Here's the drawing with two shaded views (mm, measured from the low corner). I have some questions. Coordinates: 2 decimals unless noted, no trailing zeros. Order: outer loops, then holes, each group sorted by start corner. A loop starts at its lowest first (then second) coordinate and runs counter-clockwise, first axis right, second up. Notation, with made-up numbers: (16.5, -34) -> (23.5, -34) arc R28 ccw to (23.5, 1) -> close; hole circle Ø10 at (31.5, 1.5). An arc over 180 degrees is marked (long way). Write item = value, one per line.
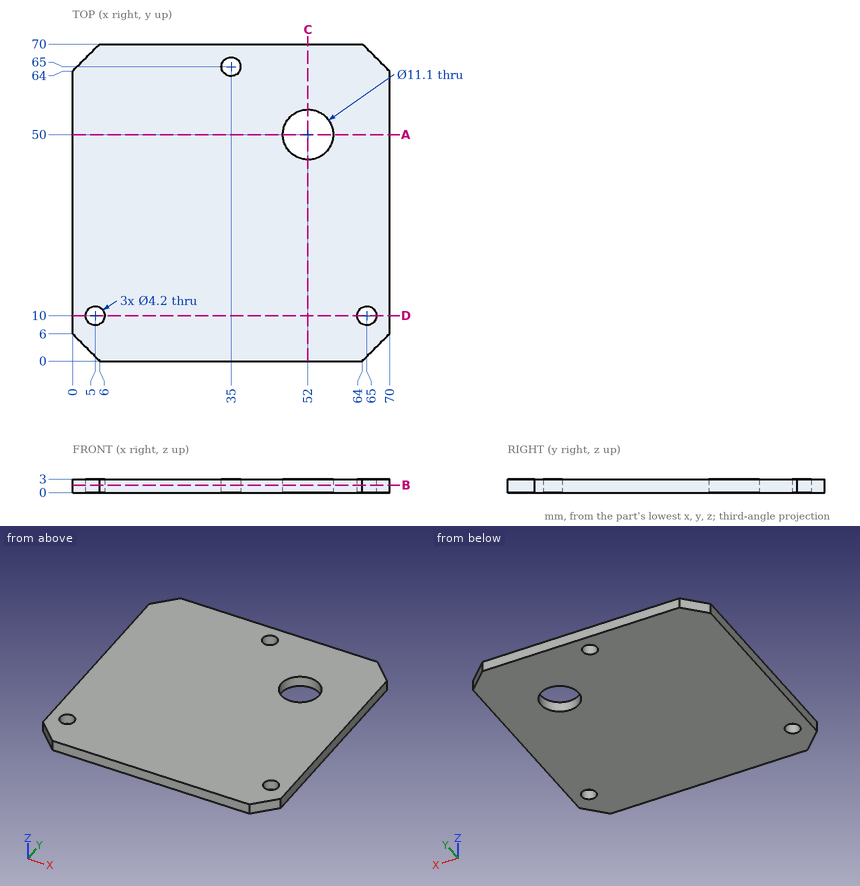
Item 1: I want a section at A-A, the plane y = 50. Please give me the cut outline in (x, z).
A:
outline = (0, 0) -> (46.45, 0) -> (46.45, 3) -> (0, 3) -> close; (57.55, 0) -> (70, 0) -> (70, 3) -> (57.55, 3) -> close
Item 2: I want a section at D-D, the plane y = 10. Please give me the cut outline in (x, z).
A:
outline = (0, 0) -> (2.9, 0) -> (2.9, 3) -> (0, 3) -> close; (7.1, 0) -> (62.9, 0) -> (62.9, 3) -> (7.1, 3) -> close; (67.1, 0) -> (70, 0) -> (70, 3) -> (67.1, 3) -> close
Item 3: I'm going to push flat-ended pins straight in: P1, Ø2.5, axis at x = 65, y = 10, coming from the +Z side; P2, Ø6.5, axis at x = 35, y = 65, coming from the +Z side. Where does each tip first touch, or does it pass through?
A:
P1 = through
P2 = 3
Item 4: I want a section at B-B, the plane z = 1.65. Please give me the cut outline in (x, y).
A:
outline = (0, 6) -> (6, 0) -> (64, 0) -> (70, 6) -> (70, 64) -> (64, 70) -> (6, 70) -> (0, 64) -> close; hole circle Ø4.2 at (5, 10); hole circle Ø4.2 at (35, 65); hole circle Ø11.1 at (52, 50); hole circle Ø4.2 at (65, 10)
Item 5: If I drill on probe 1 along X at (y, z) = (11, 1.7); probe 2 along X at (y, z) = (66, 2.1); probe 3 along Y at (x, z) = (57, 1.95), over which ranges is the centre line in solid material (lowest first)?
A:
probe_1 = 0 to 3.15, 6.85 to 63.15, 66.85 to 70
probe_2 = 2 to 33.15, 36.85 to 68
probe_3 = 0 to 47.59, 52.41 to 70
Item 6: I want a section at C-C, the plane x = 52. Please give me the cut outline in (y, z), plus the area to 3 significant figures.
A:
outline = (0, 0) -> (44.45, 0) -> (44.45, 3) -> (0, 3) -> close; (55.55, 0) -> (70, 0) -> (70, 3) -> (55.55, 3) -> close
area = 177 mm2
